Verification items for the finished model (mm, model axes). Face numbers are marked on the shaded views. A direction names the side the tool comes from. Round coordinates to 2 decimals unless told otherwise and drop trailing zeros. Loops run counter-clockwise (first coordinate to the right, second up) from the corner with the lowest first, then second, coordinate; pieces in that order, holes last. Notation, with made-up numbers: (-10, 42.5) - (42, 42.5) arc R20 ccw to (42, 53.5) - close; hole circle Ø2 at (-30.5, -37.5). An arc over 180 degrees is marked (long way). Use CSV: the item, a comma, the result in double quotes.
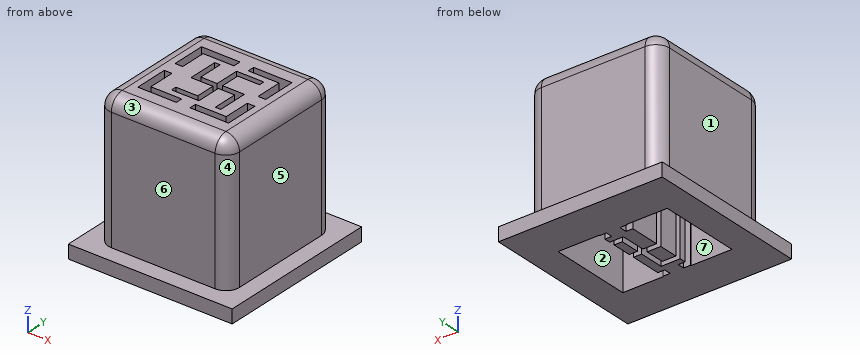
```python
from build123d import *

# Parameters (mm, degrees)
SKETCH_W        = 9.6
SKETCH_H        = 9.6
PAD_DEPTH       = 10
SKETCH002_W     = 12
SKETCH002_H     = 12
PAD001_DEPTH    = 1
SKETCH003_W     = 3
SKETCH003_H     = 6
POCKET_DEPTH    = 9
SKETCH004_W     = 3
SKETCH004_H     = 6
POCKET001_DEPTH = 9
POCKET002_DEPTH = 11.001
POCKET003_DEPTH = 11.001
POCKET004_DEPTH = 11.001
POCKET005_DEPTH = 11.001
FILLET_R        = 1
POCKET006_DEPTH = 11.001


with BuildPart() as part:
    # Sketch → Pad (new body)
    with BuildSketch(Plane.XY):
        Rectangle(SKETCH_W, SKETCH_H)
    extrude(amount=PAD_DEPTH)

    # Sketch002 → Pad001 (join)
    with BuildSketch(Plane(origin=(0, 0, 0), x_dir=(1, 0, 0), z_dir=(0, 0, -1))):
        Rectangle(SKETCH002_W, SKETCH002_H)
    extrude(amount=PAD001_DEPTH)

    # Sketch003 → Pocket (cut)
    with BuildSketch(Plane(origin=(0, 0, -2), x_dir=(1, 0, 0), z_dir=(0, 0, -1))):
        with Locations((-2.5, 0)):
            Rectangle(SKETCH003_W, SKETCH003_H)
    extrude(amount=-POCKET_DEPTH, mode=Mode.SUBTRACT)

    # Sketch004 → Pocket001 (cut)
    with BuildSketch(Plane(origin=(0, 0, -2), x_dir=(1, 0, 0), z_dir=(0, 0, -1))):
        with Locations((2.5, 0)):
            Rectangle(SKETCH004_W, SKETCH004_H)
    extrude(amount=-POCKET001_DEPTH, mode=Mode.SUBTRACT)

    # Sketch001 → Pocket002 (cut, through all)
    with BuildSketch(Plane.XY.offset(10)):
        Polygon((3.32, -0.5), (3.32, -2.95), (0.5, -2.95), (0.5, -2.45), (2.76, -2.45), (2.76, -0.5), align=None)
    extrude(amount=-POCKET002_DEPTH, mode=Mode.SUBTRACT)

    # Sketch005 → Pocket003 (cut, through all)
    with BuildSketch(Plane.XY.offset(10)):
        Polygon((-3.32, -0.5), (-3.32, -2.95), (-0.5, -2.95), (-0.5, -2.45), (-2.76, -2.45), (-2.76, -0.5), align=None)
    extrude(amount=-POCKET003_DEPTH, mode=Mode.SUBTRACT)

    # Sketch007 → Pocket004 (cut, through all)
    with BuildSketch(Plane.XY.offset(10)):
        Polygon((-2.76, 0.5), (-3.32, 0.5), (-3.32, 2.95), (-0.5, 2.95), (-0.5, 2.39), (-2.76, 2.39), align=None)
    extrude(amount=-POCKET004_DEPTH, mode=Mode.SUBTRACT)

    # Sketch006 → Pocket005 (cut, through all)
    with BuildSketch(Plane.XY.offset(10)):
        Polygon((0.5, 2.95), (3.32, 2.95), (3.32, 0.5), (2.76, 0.5), (2.76, 2.45), (0.5, 2.45), align=None)
    extrude(amount=-POCKET005_DEPTH, mode=Mode.SUBTRACT)

    # Fillet
    fillet_edges = [part.edges().sort_by_distance(p)[0] for p in [
        (0, 4.8, 10),
        (4.8, 0, 10),
        (0, -4.8, 10),
        (4.8, -4.8, 5),
        (4.8, 4.8, 5),
        (-4.8, 0, 10),
        (-4.8, -4.8, 5),
        (-4.8, 4.8, 5),
    ]]
    fillet(fillet_edges, radius=FILLET_R)

    # Sketch008 (on Face23 of Fillet) → Pocket006 (cut, through all)
    with BuildSketch(Plane.XY.offset(10)):
        Polygon((0.4, -0.2), (0.4, -2), (-1.6, -2), (-1.6, -1.598578), (0, -1.598578), (0, -0.2), (-1.6, -0.2), (-1.6, 2), (-1.2, 2), (-1.2, 0.2), (0, 0.2), (0, 2), (2, 2), (2, 1.6), (0.4, 1.6), (0.4, 0.2), (2, 0.2), (2, -2), (1.6, -2), (1.6, -0.2), align=None)
    extrude(amount=-POCKET006_DEPTH, mode=Mode.SUBTRACT)


solid = part.part
```
1) Cross-section at B-B, the plane y = -2.75. Record the cut outline in (x, z).
Returned:
outline,"(-6, -1) - (-4, -1) - (-4, 7) - (-3.32, 7) - (-3.32, 10) - (-3.8, 10) arc R1 ccw to (-4.8, 9) - (-4.8, 0) - (-6, 0) - close; (-0.5, -1) - (0.5, -1) - (0.5, 10) - (-0.5, 10) - close; (3.32, 7) - (4, 7) - (4, -1) - (6, -1) - (6, 0) - (4.8, 0) - (4.8, 9) arc R1 ccw to (3.8, 10) - (3.32, 10) - close"
2) Cross-section at D-D, the plane z = 3.5. Count the separate pieces of the cut face and the enclosed holes in it, then the cut area to 3 significant figures.
Returned:
separate pieces,"3"
enclosed holes,"1"
area,"51.4 mm²"
3) Cross-section at C-C, the plane x = 2.25. Record the cut outline in (y, z).
Returned:
outline,"(-6, -1) - (-3, -1) - (-3, 7) - (-2.95, 7) - (-2.95, 10) - (-3.8, 10) arc R1 ccw to (-4.8, 9) - (-4.8, 0) - (-6, 0) - close; (-2.45, 7) - (2.45, 7) - (2.45, 10) - (-2.45, 10) - close; (2.95, 7) - (3, 7) - (3, -1) - (6, -1) - (6, 0) - (4.8, 0) - (4.8, 9) arc R1 ccw to (3.8, 10) - (2.95, 10) - close"
4) Cross-section at A-A, the plane x = 0.75. Record the cut outline in (y, z).
Returned:
outline,"(-6, -1) - (-2.95, -1) - (-2.95, 10) - (-3.8, 10) arc R1 ccw to (-4.8, 9) - (-4.8, 0) - (-6, 0) - close; (-2.45, -1) - (-0.2, -1) - (-0.2, 10) - (-2.45, 10) - close; (0.2, -1) - (1.6, -1) - (1.6, 10) - (0.2, 10) - close; (2, -1) - (2.45, -1) - (2.45, 10) - (2, 10) - close; (2.95, -1) - (6, -1) - (6, 0) - (4.8, 0) - (4.8, 9) arc R1 ccw to (3.8, 10) - (2.95, 10) - close"
5) Mould release check, pull along Y, two halves, no side actions. Record for the marked faces 1, 2 and 3: +Y half, -Y half, draft (parallel to the pull), parting line (faces both ways), or undercut.
Returned:
face 1,"draft"
face 2,"undercut"
face 3,"-Y half"
6) Gauge pin test, flat ends, axial feed: pin 1 Ø3 at (x, z) = (4.5, 8.5) entering from -Y; pin 2 Ø2.5 at (y, z) = (0.5, 9) entering from +X; pin 3 Ø0.5 at (x, z) = (-1, 4.5) entering from +Y. Record the tip position at first contact, or that the pin passes through.
Returned:
pin 1,"stops at y = -4.8"
pin 2,"stops at x = 4.8"
pin 3,"stops at y = 4.8"
7) Access from +Z, -Z, +X, -X, +Y, -Y to the whole of each face (thin tool, end or side, straight path). Record for the marked faces 4, 5, 6 and 7.
Returned:
face 4,"+Z, +X, -Y"
face 5,"+Z, +X, +Y, -Y"
face 6,"+Z, +X, -X, -Y"
face 7,"-Z"
8) Thickness scan on probe 1 along X at (y, z) = (1.5, 9); probe 2 along X at (y, z) = (1.25, 2.75); probe 3 along X at (y, z) = (-0.25, -0.5). Record the ranges inside material, lowest first. Write a range as [from, to].
Returned:
probe 1,"x = [-4.8, -3.32], [-2.76, -1.6], [-1.2, 0], [0.4, 2.76], [3.32, 4.8]"
probe 2,"x = [-4.8, -4], [-1, 0], [0.4, 1], [4, 4.8]"
probe 3,"x = [-6, -4], [-1, 0], [0.4, 1], [4, 6]"
